from build123d import *

# Parameters (mm, degrees)
SKETCH1_W                  = 63.5
SKETCH1_H                  = 6.35
BOSS_EXTRUDE1_DEPTH        = 76.2
F_10_CLEARANCE_HOLE1_D     = 5.1054
F_10_CLEARANCE_HOLE1_DEPTH = 9.652
F_10_CLEARANCE_HOLE1_TIP   = 1.533816902


with BuildPart() as part:
    # Sketch1 → Boss-Extrude1 (new, symmetric)
    with BuildSketch(Plane(origin=(0, 0, 0), x_dir=(0, 0, -1), z_dir=(1, 0, 0))):
        Rectangle(SKETCH1_W, SKETCH1_H)
    extrude(amount=BOSS_EXTRUDE1_DEPTH, both=True)

    # #10 Clearance Hole1
    with Locations(Plane(origin=(0, 3.175, 0), x_dir=(1, 0, 0), z_dir=(0, 1, 0))):
        with Locations((-4.7625, 22.225), (36.5125, -22.225), (-4.7625, -22.225), (36.5125, 22.225)):
            Hole(F_10_CLEARANCE_HOLE1_D / 2, depth=F_10_CLEARANCE_HOLE1_DEPTH)
            with Locations((0, 0, -(F_10_CLEARANCE_HOLE1_DEPTH + F_10_CLEARANCE_HOLE1_TIP / 2))):  # 118° drill point
                Cone(0, F_10_CLEARANCE_HOLE1_D / 2, F_10_CLEARANCE_HOLE1_TIP, mode=Mode.SUBTRACT)


solid = part.part
Check sheet for the modelled part. Datum: model origin and axes. Units: mm. Round coordinates to 2 decimals unless told otherwise and drop trailing zeros. Return JSON: item names as keys, results as strings.
Q1. Draft check along Z on faces 1 (the cylindrical face through (34.078, -0.044, 21.458)), 2 (the flat face through (1, 0, -31.75)), 3 (the flat face through (1, 0, 31.75)), 4 (the flat face through (76.2, 0, 0)). Enter one of: released by +Z, released by -Z, zero draft, split by the parting line, or undercut.
Returned:
{"face 1": "undercut", "face 2": "released by -Z", "face 3": "released by +Z", "face 4": "zero draft"}
Q2. Scan lines: L1, parallel to X at y = 1.75, z = -24; L2, parallel to X at y = 2.75, z = 20.5; L3, parallel to Z at x = 36, y = -2.5. Record each from-to range of solid material in increasing order. Write a range as from..to.
Returned:
{"L1": "x = -76.2..-6.6, -2.93..34.68, 38.35..76.2", "L2": "x = -76.2..-6.64, -2.88..34.63, 38.39..76.2", "L3": "z = -31.75..-24.73, -19.72..19.72, 24.73..31.75"}
Q3. Depth check by flat-ended pin: P1, Ø3, axis at x = 36.51, z = -22.22, coming from the -Y side. Enter the tip coordinate at first touch or a pass-through.
Returned:
{"P1": "passes through"}
